```python
from build123d import *

# Parameters (mm, degrees)
SKETCH1_W          = 825.5
SKETCH1_H          = 254
BASE_FLANGE1_DEPTH = 4.7625
SKETCH6_W          = 38.1
SKETCH6_H          = 76.2
SKETCH6_W_2        = 241.3
SKETCH6_H_2        = 101.6
SKETCH6_W_3        = 50.8
CUT_EXTRUDE1_DEPTH = 432.872948801
SKETCH7_W          = 177.8
SKETCH7_H          = 50.8
SKETCH7_W_2        = 120.65
SKETCH7_H_2        = 25.4
CUT_EXTRUDE2_DEPTH = 432.872948801
CUT_EXTRUDE3_DEPTH = 432.872948801


# Sheet-metal steps are written as plain solids
with BuildPart() as part:
    # Sketch1 → Base-Flange1 (new body)
    with BuildSketch(Plane(origin=(0, 0, 0), x_dir=(1, 0, 0), z_dir=(0, 1, 0))):
        Rectangle(SKETCH1_W, SKETCH1_H)
    extrude(amount=-BASE_FLANGE1_DEPTH)

    # Sketch6 → Cut-Extrude1 (cut, through all)
    with BuildSketch(Plane(origin=(0, 0, 0), x_dir=(1, 0, 0), z_dir=(0, 1, 0))):
        with Locations((0, 127)):
            Rectangle(SKETCH6_W, SKETCH6_H)
        with Locations((-412.75, 50.8)):
            Rectangle(SKETCH6_W_2, SKETCH6_H_2)
        with Locations((412.75, 50.8)):
            Rectangle(SKETCH6_W_2, SKETCH6_H_2)
        with Locations((-69.85, 127)):
            Rectangle(SKETCH6_W_3, SKETCH6_H_2)
    extrude(amount=-CUT_EXTRUDE1_DEPTH, mode=Mode.SUBTRACT)

    # Sketch7 → Cut-Extrude2 (cut, through all)
    with BuildSketch(Plane(origin=(0, 0, 0), x_dir=(1, 0, 0), z_dir=(0, 1, 0))):
        with Locations((-323.85, 101.6)):
            Rectangle(SKETCH7_W, SKETCH7_H)
        with Locations((352.425, 114.3)):
            Rectangle(SKETCH7_W_2, SKETCH7_H_2)
    extrude(amount=-CUT_EXTRUDE2_DEPTH, mode=Mode.SUBTRACT)

    # Sketch8 → Cut-Extrude3 (cut, through all)
    with BuildSketch(Plane(origin=(0, 0, 0), x_dir=(1, 0, 0), z_dir=(0, 1, 0))):
        Polygon((341.654432116, -82.55), (374.65, -101.6), (374.65, -63.5), align=None)
        Polygon((323.85, -101.6), (323.85, -63.5), (290.854432116, -82.55), align=None)
        Polygon((273.05, -101.6), (273.05, -63.5), (240.054432116, -82.55), align=None)
        Polygon((222.25, -101.6), (222.25, -63.5), (189.254432116, -82.55), align=None)
        Polygon((171.45, -101.6), (171.45, -63.5), (138.454432116, -82.55), align=None)
        Polygon((120.65, -101.6), (120.65, -63.5), (87.654432116, -82.55), align=None)
        Polygon((69.85, -101.6), (69.85, -63.5), (36.854432116, -82.55), align=None)
        Polygon((-36.854432116, -82.55), (-69.85, -101.6), (-69.85, -63.5), align=None)
        Polygon((-87.654432116, -82.55), (-120.65, -101.6), (-120.65, -63.5), align=None)
        Polygon((-138.454432116, -82.55), (-171.45, -101.6), (-171.45, -63.5), align=None)
        Polygon((-189.254432116, -82.55), (-222.25, -101.6), (-222.25, -63.5), align=None)
        Polygon((-240.054432116, -82.55), (-273.05, -101.6), (-273.05, -63.5), align=None)
        Polygon((-290.854432116, -82.55), (-323.85, -101.6), (-323.85, -63.5), align=None)
        Polygon((-374.65, -63.5), (-341.654432116, -82.55), (-374.65, -101.6), align=None)
    extrude(amount=-CUT_EXTRUDE3_DEPTH, mode=Mode.SUBTRACT)


solid = part.part
```
Geometry: final body of the model. Coordinates: model frame, mm. A direction names the side the tool comes from. Give positions to 0.01 mm unless a question says otherwise; leave off trailing zeros. Order: outer loops, then holes, each group sorted by start corner. A loop starts at its lowest first (then second) coordinate and runs counter-clockwise, first axis right, second up. Notation, with made-up numbers: M -9,-31.75 L 34,-31.75 A30 ccw 34,4.25 Z; hole C 39.5,24.25 d4. An arc over 180 degrees is marked long. Answer as CSV lines item,"result". Start each with the question number.
1) Cut plane B-B (x = 300.5). Output: boundary loops of the cut face in (y, z).
2) Set-up query: faces 3 (the flat face through (-6, 0, -2)), 4 (the flat face through (-307.12, -2.35, 91.94)). Return all of +Z, -Z, +X, -X, +Y, -Y with unobstructed straight access to the full face (end or side cutting, diameter ignored); none if empty.
3) First-contact query: P1, Ø2.5, axis at y = -3, z = -68, coming from the +X side; P2, Ø1.4, axis at y = -3, z = -105.5, coming from the -X side; P3, Ø2.5, axis at x = -60.5, y = -3, coming from the -Z side. Flat tips, straight axial feed; report the tip coordinate or a pass-through.
4) Mould query, pull axis X, two halves, no side actions, for faces 1 (the flat face through (-154.72, -2.35, 91.94)), 2 (the flat face through (-6, -4.762, -2)). Classes: +X half, -X half, draft (parallel to the pull), parting line (faces both ways), or undercut.
5) Cut plane A-A (z = -97). Output: boundary loops of the cut face in (x, y), then the cut area to 3 significant figures.
6) Cut plane C-C (y = -2.6). State how many separate pieces and enclosed holes the cut face has, then the cut area to 3 significant figures.
7) Cut plane D-D (z = -15). Output: boundary loops of the cut face in (x, y).
8) Line query: line 1 (X direction, y = -2.75, z = -95); line 2 (Z direction, x = 374.5, y = -4.25); line 3 (X direction, y = -1.8, z = -88.5). Output: solid intervals per line, ascending. Write a range as from..to.
Findings below:
1,outline,"M -4.76,0 L 0,0 L 0,76.98 L -4.76,76.98 Z; M -4.76,88.12 L 0,88.12 L 0,127 L -4.76,127 Z"
2,face 3,"+Z, -Z, +X, -X, +Y"
2,face 4,"+Y, -Y"
3,P1,"stops at x = 292.1"
3,P2,"stops at x = -234.95"
3,P3,"stops at z = -76.2"
4,face 1,"undercut"
4,face 2,"draft"
5,outline,"M -234.95,-4.76 L -95.25,-4.76 L -95.25,0 L -234.95,0 Z; M -44.45,-4.76 L -19.05,-4.76 L -19.05,0 L -44.45,0 Z; M 19.05,-4.76 L 292.1,-4.76 L 292.1,0 L 19.05,0 Z"
5,area,"2,090 mm²"
6,separate pieces,"1"
6,enclosed holes,"14"
6,area,"163,000 mm²"
7,outline,"M -292.1,-4.76 L 292.1,-4.76 L 292.1,0 L -292.1,0 Z"
8,line 1,"x = -234.95..-95.25, -44.45..-19.05, 19.05..292.1"
8,line 2,"z = 0..63.59, 101.51..127"
8,line 3,"x = -234.95..-95.25, -44.45..292.1"
